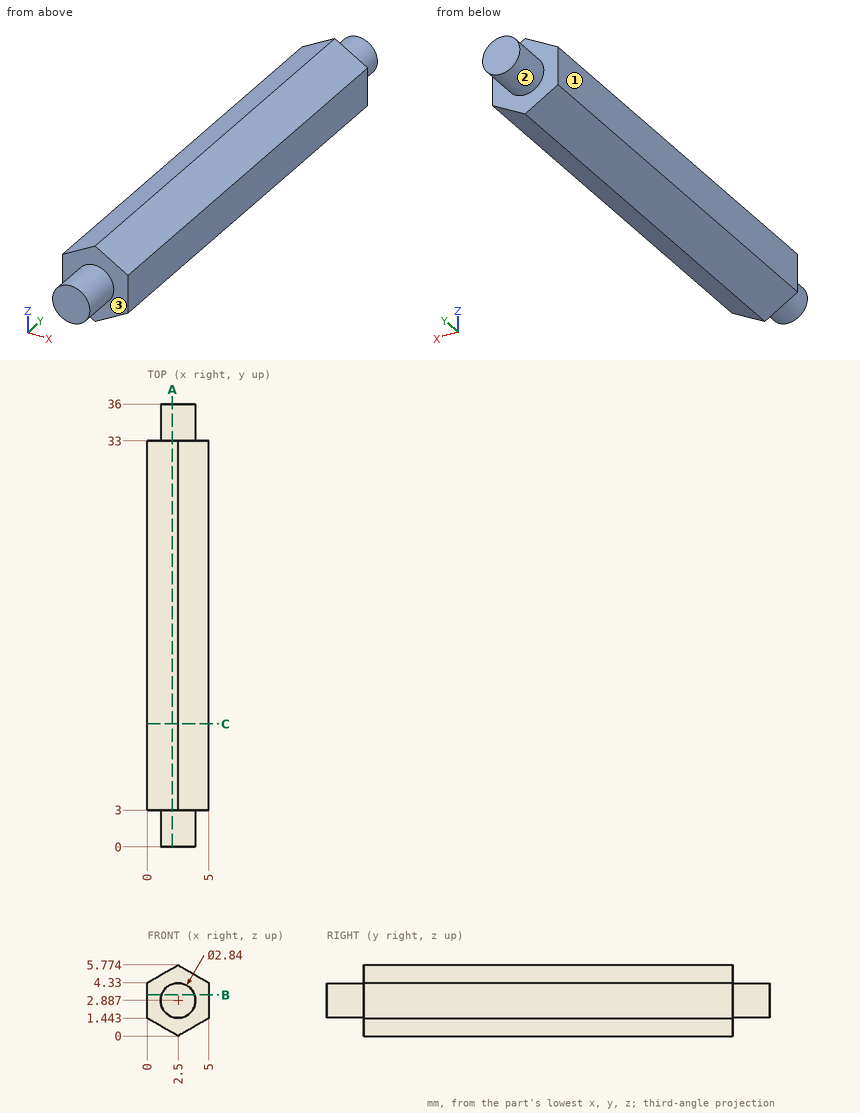
Study the drawing (mm; zero at the part's minimum x, y, z) and answer. A direction names the side the tool comes from. Coordinates: 2 decimals unless noted, no trailing zeros. Write each loop counter-clockwise with the first axis right and the second up, starting at its lowest first coordinate (ties: lowest second). Pieces come first, ordered by that corner, then holes. Notation, with made-up numbers: (42, -19) - (91, -19) arc R17 ccw to (91, 2) - close; hole circle Ø3 at (58, 71). An arc over 180 degrees is marked (long way). Return JSON: item names as keys, results as strings. Group by question number.
1. Given pin 1 (1 mm diameter, centred on x = 4, z = 1, fed in from +Y), flat-ended and moving along its own axis, determine where the tip first touches the part or whether it passes through.
2. A cutting plane is placed at C-C, the plane y = 10. Determine the outline of the cut face in (x, z).
3. Which of the six approach directions +Z, -Z, +X, -X, +Y, -Y give full straight-line access (tool end or side, diameter ignored) to the marked faces 1, 2 and 3?
4. Straight lines are drawn through the part: L1, parallel to Y at x = 3, z = 1.05; L2, parallel to X at y = 13, z = 1 (1 decimal); L3, parallel to Z at x = 1.7, y = 22. For each, find the intervals that lie inside material, in ascending order.
5. A cutting plane is placed at A-A, the plane x = 2.05. Determine the outline of the cut face in (y, z).
6. A cutting plane is placed at B-B, the plane z = 3.35. Determine the outline of the cut face in (x, y).
Ans:
{
 "1": {"pin 1": "y = 33"},
 "2": {"outline": "(0, 1.44) - (2.5, 0) - (5, 1.44) - (5, 4.33) - (2.5, 5.77) - (0, 4.33) - close"},
 "3": {"face 1": "+Z, -Z, -X, +Y, -Y", "face 2": "+Y", "face 3": "-Y"},
 "4": {"L1": "3 to 33", "L2": "0.8 to 4.2", "L3": "0.46 to 5.31"},
 "5": {"outline": "(0, 1.54) - (3, 1.54) - (3, 0.26) - (33, 0.26) - (33, 1.54) - (36, 1.54) - (36, 4.23) - (33, 4.23) - (33, 5.51) - (3, 5.51) - (3, 4.23) - (0, 4.23) - close"},
 "6": {"outline": "(0, 3) - (1.16, 3) - (1.16, 0) - (3.84, 0) - (3.84, 3) - (5, 3) - (5, 33) - (3.84, 33) - (3.84, 36) - (1.16, 36) - (1.16, 33) - (0, 33) - close"}
}
